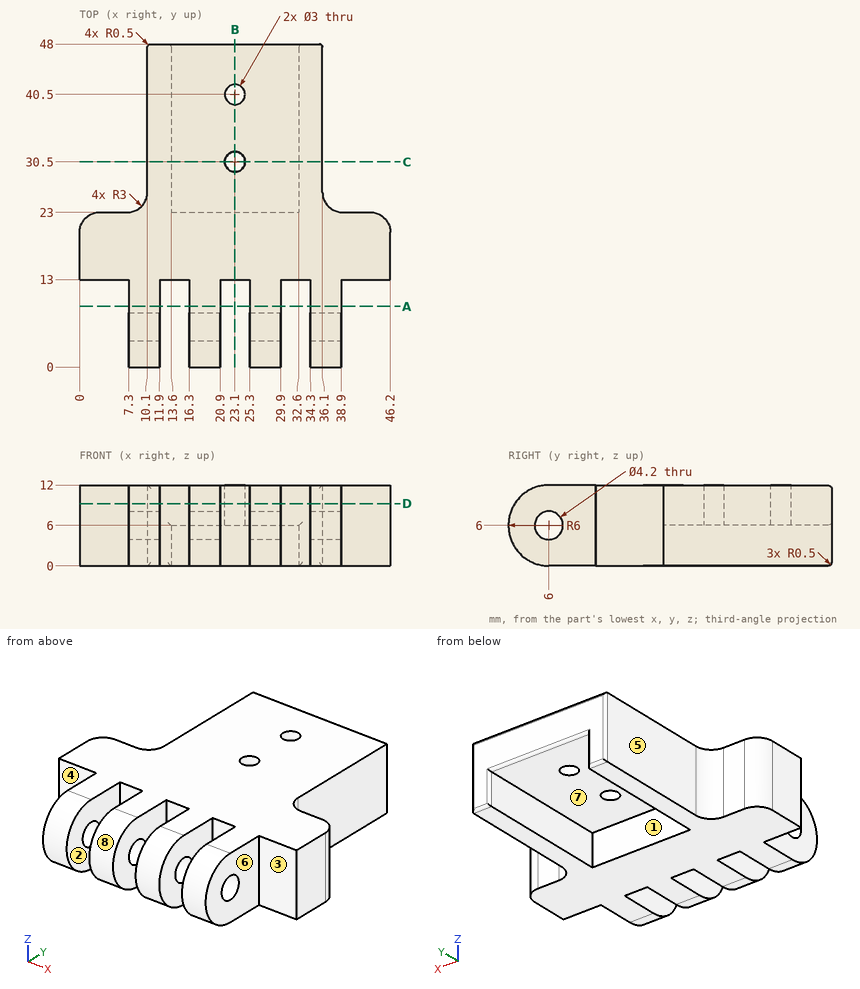
Answer from the drawing. Dimensions are ordinates in mm from the lowest x, y and z of the part. A direction names the side the tool comes from. Round coordinates to 2 decimals unless told otherwise and drop trailing zeros. Loops run counter-clockwise (first coordinate to the right, second up) from the corner with the lowest first, then second, coordinate; pieces in that order, holes last. Notation, with made-up numbers: (79.25, -36.5) - (113.25, -36.5) arc R35 ccw to (113.25, 2.5) - close; hole circle Ø1 at (49.5, 35.5). An arc over 180 degrees is marked (long way). One line per item, written item: value.
Q1. Straight lines are drawn through the part: probe 1 along Y at (x, z) = (23.1, 8.35); probe 2 along X at (y, z) = (27.5, 2.75); probe 3 along X at (y, z) = (42.5, 7.75). For each, find the intervals that lie inside material, in ascending order.
Check values:
probe 1: 13 to 29, 32 to 39, 42 to 48
probe 2: 10.1 to 13.6, 32.6 to 36.1
probe 3: 10.1 to 36.1
Q2. For the marked faces 1, 2, 3, 4 and 5, determine the directions among +Z, -Z, +X, -X, +Y, -Y from which every point of the face is accessible in a straight line to the end or side of a thin tool.
Check values:
face 1: -Z, +Y
face 2: +Z, -Z, -Y
face 3: +Z, -Z, +X, -Y
face 4: +Z, -Z, -X, -Y
face 5: +Z, -Z, -X, +Y
Q3. Find section C-C on y = 30.5. Give the vertices of the cut face in (x, z).
Check values:
outline: (10.1, 0) - (13.6, 0) - (13.6, 6) - (21.6, 6) - (21.6, 12) - (10.1, 12) - close; (24.6, 6) - (32.6, 6) - (32.6, 0) - (36.1, 0) - (36.1, 12) - (24.6, 12) - close
Q4. Find section D-D on z = 9.25. State how many separate pieces and enclosed holes the cut face has, and give its area (3 significant figures).
Check values:
separate pieces: 1
enclosed holes: 2
area: 1,320 mm2
Q5. Find section B-B on x = 23.1. Give the vertices of the cut face in (y, z).
Check values:
outline: (13, 0) - (23, 0) - (23, 6) - (29, 6) - (29, 12) - (13, 12) - close; (32, 6) - (39, 6) - (39, 12) - (32, 12) - close; (42, 6) - (47.5, 6) arc R0.5 ccw to (48, 6.5) - (48, 11.5) arc R0.5 ccw to (47.5, 12) - (42, 12) - close
Q6. The mould has two halves that part along X. Classify the marked faces 6, 7 and 8: +X half, -X half, draft (parallel to the pull), parting line (faces both ways), or undercut.
Check values:
face 6: +X half
face 7: undercut
face 8: draft
Q7. Each of these flat-tipped pins is pushed along its axis until it touches: pin 1 Ø5 at (x, z) = (23, 4) entering from -Y; pin 2 Ø3.5 at (y, z) = (4, 5) entering from +X; pin 3 Ø1.2 at (x, z) = (5.5, 3.5) entering from +Y. Where does it stop, or does it pass through?
Check values:
pin 1: y = 0.03
pin 2: x = 38.9
pin 3: y = 23
Q8. Find section A-A on y = 9. Give the vertices of the cut face in (x, z).
Check values:
outline: (7.3, 0) - (11.9, 0) - (11.9, 12) - (7.3, 12) - close; (16.3, 0) - (20.9, 0) - (20.9, 12) - (16.3, 12) - close; (25.3, 0) - (29.9, 0) - (29.9, 12) - (25.3, 12) - close; (34.3, 0) - (38.9, 0) - (38.9, 12) - (34.3, 12) - close
